Verification items for the finished model (mm, model axes). A direction names the side the tool comes from. Coordinates: 2 decimals unless noted, no trailing zeros. Write each loop counter-clockwise with the first axis right and the second up, starting at its lowest first coordinate (ties: lowest second). Pieces come first, ordered by that corner, then holes. Notation, with made-up numbers: (0, 81.25) -> (26, 81.25) arc R21 cw to (26, 117.25) -> close; hole circle Ø9 at (-12.5, 43.5). An arc over 180 degrees is marked (long way). Use a Markdown table: item, result. Add a question column.
from build123d import *

# Parameters (mm, degrees)
EXTRUDE_1_DEPTH = 2
SKETCH_3_W      = 90
SKETCH_3_H      = 2
EXTRUDE_2_DEPTH = 10


with BuildPart() as part:
    # 草图2 → 凸台-拉伸1 (new body)
    with BuildSketch(Plane(origin=(0, 0, 0), x_dir=(1, 0, 0), z_dir=(0, 1, 0))):
        Polygon((-0.5, 69.85106383), (-45, 69.85106383), (-45, -64.14893617), (45, -64.14893617), (45, 69.85106383), align=None)
    extrude(amount=EXTRUDE_1_DEPTH)

    # 草图3 → 凸台-拉伸2 (add)
    with BuildSketch(Plane(origin=(0, 0, 0), x_dir=(1, 0, 0), z_dir=(0, 1, 0))):
        with Locations((0, 68.85106383)):
            Rectangle(SKETCH_3_W, SKETCH_3_H)
        with Locations((0, -63.14893617)):
            Rectangle(SKETCH_3_W, SKETCH_3_H)
    extrude(amount=-EXTRUDE_2_DEPTH)


solid = part.part
1) Cross-section at A-A on y = -1.5. Record the boundary of the cut face in (x, z).
2) Cross-section at C-C on z = -60. Record the boundary of the cut face in (x, y), then the cut area to 3 significant figures.
3) Set-up check for faces 4 (the face through (45, 1, -3)), 5 (the face through (-1, 0, -4)): record each of +Z, -Z, +X, -X, +Y, -Y from which the full face is reachable in a straight line by a thin tool's end or side.
4) Thickness scan on L1, parallel to Z at x = 14, y = -7; L2, parallel to Y at x = -17, z = -49.5. Record the ranges inside material, lowest first.
5) Release check for a two-part mould opening along Z. For faces 1 (the face through (-1, -4, -69.851)), 2 (the face through (-1, -5, -67.851)), 3 (the face through (-45, 1, -3)) record: released by +Z, released by -Z, zero draft, split by the parting line, or undercut.
6) Cross-section at B-B on x = 32. Record the boundary of the cut face in (y, z).
Returned:
| question | item | result |
|---|---|---|
| 1 | outline | (-45, -69.85) -> (45, -69.85) -> (45, -67.85) -> (-45, -67.85) -> close; (-45, 62.15) -> (45, 62.15) -> (45, 64.15) -> (-45, 64.15) -> close |
| 2 | outline | (-45, 0) -> (45, 0) -> (45, 2) -> (-45, 2) -> close |
| 2 | area | 180 mm² |
| 3 | face 4 | +Z, -Z, +X, +Y, -Y |
| 3 | face 5 | +X, -X, -Y |
| 4 | L1 | z = -69.85 to -67.85, 62.15 to 64.15 |
| 4 | L2 | y = 0 to 2 |
| 5 | face 1 | released by -Z |
| 5 | face 2 | undercut |
| 5 | face 3 | zero draft |
| 6 | outline | (-10, -69.85) -> (2, -69.85) -> (2, 64.15) -> (-10, 64.15) -> (-10, 62.15) -> (0, 62.15) -> (0, -67.85) -> (-10, -67.85) -> close |
